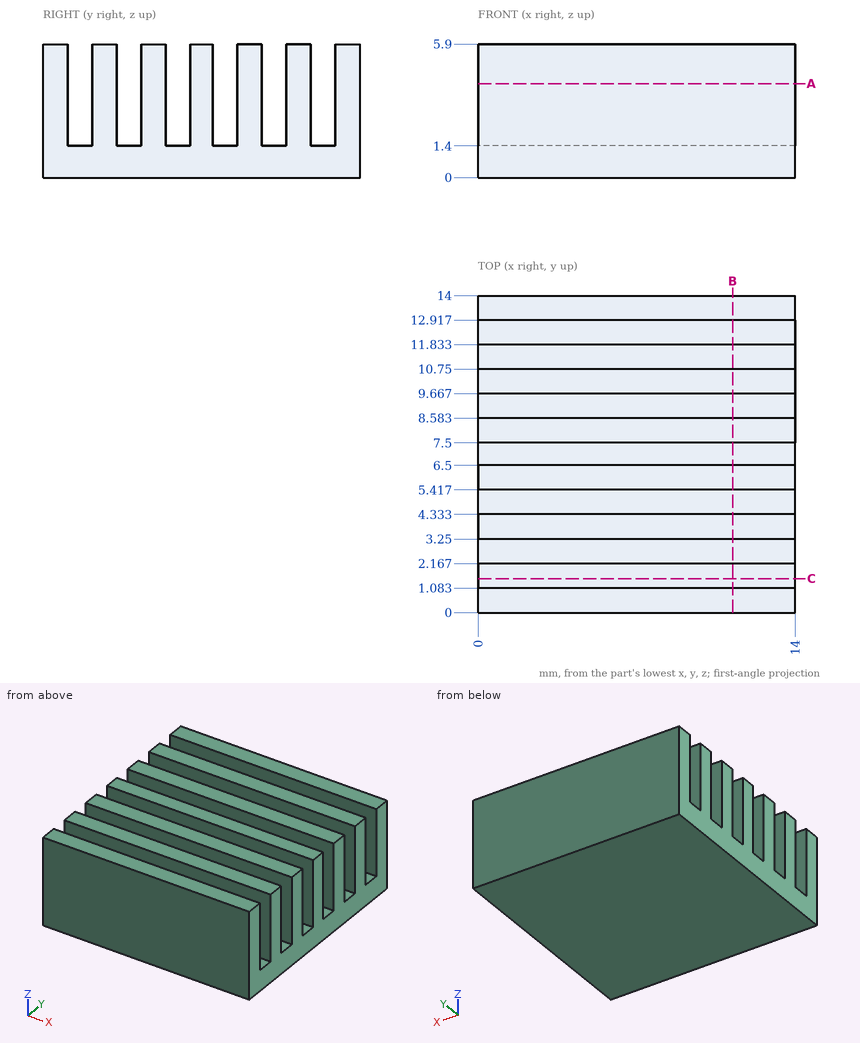
Part print with two shaded views. Sizes in mm from the minimum x, y, z corner. Round coordinates to 2 decimals unless told otherwise and drop trailing zeros. Order: outer loops, then holes, each group sorted by start corner. A loop starts at its lowest first (then second) coordinate and runs counter-clockwise, first axis right, second up.
(1) Drill centre line: line 1 (Z direction, x = 3.25, y = 12.75). Where is it in solid material? Low to high.
(2) Band-saw the part on C-C (y = 1.5). List the corners of the cut face in (x, z), then the cut area to 3 significant figures.
(3) Band-saw the part on B-B (x = 11.25). List the corners of the cut face in (y, z).
(4) Band-saw the part on A-A (z = 4.15). List the corners of the cut face in (x, y).
(5) Pin check, flat tip, straight feed: pin 1 (0.9 mm diameter, centred on x = 8.5, y = 6, fed in from +Z). Stop position of the tip, or through.
Verdict:
1. line 1: z = 0 to 1.4
2. outline: (0, 0) - (14, 0) - (14, 1.4) - (0, 1.4) - close
2. area: 19.6 mm2
3. outline: (0, 0) - (14, 0) - (14, 5.9) - (12.92, 5.9) - (12.92, 1.4) - (11.83, 1.4) - (11.83, 5.9) - (10.75, 5.9) - (10.75, 1.4) - (9.67, 1.4) - (9.67, 5.9) - (8.58, 5.9) - (8.58, 1.4) - (7.5, 1.4) - (7.5, 5.9) - (6.5, 5.9) - (6.5, 1.4) - (5.42, 1.4) - (5.42, 5.9) - (4.33, 5.9) - (4.33, 1.4) - (3.25, 1.4) - (3.25, 5.9) - (2.17, 5.9) - (2.17, 1.4) - (1.08, 1.4) - (1.08, 5.9) - (0, 5.9) - close
4. outline: (0, 0) - (14, 0) - (14, 1.08) - (0, 1.08) - close; (0, 2.17) - (14, 2.17) - (14, 3.25) - (0, 3.25) - close; (0, 4.33) - (14, 4.33) - (14, 5.42) - (0, 5.42) - close; (0, 6.5) - (14, 6.5) - (14, 7.5) - (0, 7.5) - close; (0, 8.58) - (14, 8.58) - (14, 9.67) - (0, 9.67) - close; (0, 10.75) - (14, 10.75) - (14, 11.83) - (0, 11.83) - close; (0, 12.92) - (14, 12.92) - (14, 14) - (0, 14) - close
5. pin 1: stops at z = 1.4
